Answer from the drawing. Dimensions are ordinates in mm from the lowest x, y and z of the part. A direction names the side the tool comes from. Round coordinates to 2 decimals unless told otherwise and drop trailing zeros. Loops run counter-clockwise (first coordinate to the right, second up) from the corner with the lowest first, then second, coordinate; pieces in that order, holes last. Notation, with made-up numbers: M -10.5,-4 L 26.5,-4 A21 cw 26.5,19 Z; hole C 80,23 d10. An arc over 180 degrees is marked long. One line per item, written item: value.
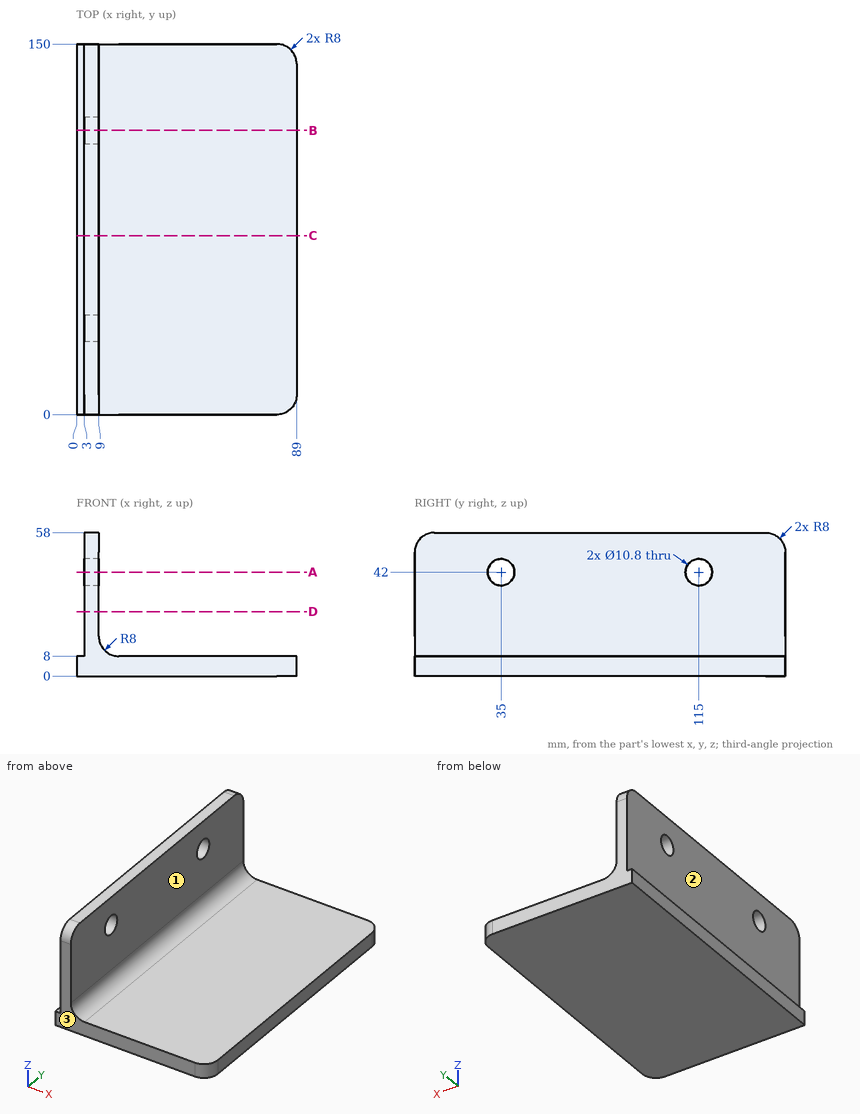
1) Find section C-C (y = 72.5). Give the vertices of the cut face in (x, z), then the cut area to 3 significant figures.
Check values:
outline: M 0,0 L 89,0 L 89,8 L 17,8 A8 cw 9,16 L 9,58 L 3,58 L 3,8 L 0,8 Z
area: 1,030 mm2
2) Find section D-D (z = 26). Give the vertices of the cut face in (x, y).
Check values:
outline: M 3,0 L 9,0 L 9,150 L 3,150 Z
3) Each of these flat-tipped pins is pushed along its axis until it touches: pin 1 (0.9 mm diameter, centred on x = 1.5, y = 106.5, fed in from +Z); pin 2 (2 mm diameter, centred on x = 53.5, y = 36.5, fed in from -Z); pin 3 (5 mm diameter, centred on y = 101, z = 12.5, fed in from -X); pin 4 (1.5 mm diameter, centred on y = 113.5, z = 11, fed in from +X). Where does it stop, or does it pass through?
Check values:
pin 1: z = 8
pin 2: z = 0
pin 3: x = 3
pin 4: x = 11.44
4) Find the intervals of material crossed by probe 1 along Y at (x, z) = (7.75, 42); probe 2 along Z at (x, y) = (7, 115); probe 3 along Z at (x, y) = (40, 106), in increasing order. Write a range as from..to.
Check values:
probe 1: 0..29.6, 40.4..109.6, 120.4..150
probe 2: 0..36.6, 47.4..58
probe 3: 0..8
5) For the marked faces 1, 2 and 3, determine the directions among +Z, -Z, +X, -X, +Y, -Y from which every point of the face is accessible in a straight line to the end or side of a thin tool.
Check values:
face 1: +Z, +X, +Y, -Y
face 2: +Z, -X, +Y, -Y
face 3: +Z, -Z, +X, -X, -Y
6) Find section A-A (z = 42). Give the vertices of the cut face in (x, y), then the cut area to 3 significant figures.
Check values:
outline: M 3,0 L 9,0 L 9,29.6 L 3,29.6 Z; M 3,40.4 L 9,40.4 L 9,109.6 L 3,109.6 Z; M 3,120.4 L 9,120.4 L 9,150 L 3,150 Z
area: 770 mm2
7) Find section B-B (y = 115). Give the vertices of the cut face in (x, z).
Check values:
outline: M 0,0 L 89,0 L 89,8 L 17,8 A8 cw 9,16 L 9,36.6 L 3,36.6 L 3,8 L 0,8 Z; M 3,47.4 L 9,47.4 L 9,58 L 3,58 Z
